```python
from build123d import *

# Parameters (mm, degrees)
ESBO_O1_R                                  = 3
RESSALTO_EXTRUS_O1_DEPTH                   = 1.5
ESBO_O2_R                                  = 2.15
RESSALTO_EXTRUS_O2_DEPTH                   = 6
BROCA_DE_ROSQUEAR_PARA_TARRAXA_DE_M3X0_5_D = 2.5
FILETE1_R                                  = 0.3


with BuildPart() as part:
    # Esboço1 → Ressalto-extrusão1 (new body)
    with BuildSketch(Plane.XY):
        with Locations((-15.341260315, 7.915210608)):
            Circle(ESBO_O1_R)
    extrude(amount=RESSALTO_EXTRUS_O1_DEPTH)

    # Esboço2 → Ressalto-extrusão2 (add)
    with BuildSketch(Plane.XY.offset(1.5)):
        with Locations((-15.341260315, 7.915210608)):
            Circle(ESBO_O2_R)
    extrude(amount=RESSALTO_EXTRUS_O2_DEPTH)

    # Broca de rosquear para tarraxa de M3x0.51 (through all)
    with Locations(Plane(origin=(0, 0, 0), x_dir=(-1, 0, 0), z_dir=(0, 0, -1))):
        with Locations((15.341260315, 7.915210608)):
            Hole(BROCA_DE_ROSQUEAR_PARA_TARRAXA_DE_M3X0_5_D / 2)

    # Filete1
    filete1_edges = [part.edges().sort_by_distance(p)[0] for p in [
        (-17.491260315, 7.915210608, 7.5),
    ]]
    fillet(filete1_edges, radius=FILETE1_R)


solid = part.part
```
The model under review builds one solid part; all positions refer to its coordinate system, in mm. A direction names the side the tool comes from. Round coordinates to 2 decimals unless told otherwise and drop trailing zeros. Loops run counter-clockwise (first coordinate to the right, second up) from the corner with the lowest first, then second, coordinate; pieces in that order, holes last. Notation, with made-up numbers: (-24.5, 84.5) -> (9.5, 84.5) arc R24 ccw to (9.5, 109.5) -> close; hole circle Ø11 at (62, 49). An arc over 180 degrees is marked (long way). Answer as a JSON object with one key per item and string values. Group by question number.
1) We need section B-B on z = 4.75. Write out the cut boundary in (x, y), then the cut area to 3 significant figures.
2) For pin 1 Ø3 at (x, z) = (-15, 3.5) entering from +Y; pin 2 Ø2 at (x, y) = (-15.34, 7.92) entering from -Z; pin 3 Ø1.5 at (x, y) = (-13, 6) entering from -Z; pin 4 Ø3 at (x, z) = (-14.5, 4) entering from -Y, all flat-tipped, find the tip position at first contact; note any pin that passes through.
3) For line 1 (Z direction, x = -14.3, y = 10.05); line 2 (X direction, y = 9, z = 3.5) (3 decimals); line 3 (Y direction, x = -15.95, z = 4.5), list the stretches that pass through material, from the lowest coordinate up. Write a range as [from, to].
4) We need section D-D on z = 1. Write out the cut boundary in (x, y), then the cut area to 3 significant figures.
5) Mouldability with a two-part tool opening along Y and no side actions: class faces 3 (the face through (-16.26, 8.76, 3.8)), 4 (the face through (-14.349, 6.008, 4.31)), 5 (the face through (-14, 7, 0)) as released by +Y, released by -Y, zero draft, split by the parting line, or undercut.
6) For faces 1 (the face through (-13, 7, 1.5)), 2 (the face through (-17, 8, 7.5)), list the 3-axis set-ups (+Z, -Z, +X, -X, +Y, -Y) from which the entire face can be reached by the end or side of a thin tool; tool diameter is ignored.
7) We need section C-C on y = 5.5. Write out the cut boundary in (x, z).
8) We need section A-A on x = -13.1. Write out the cut boundary in (y, z), then the cut area to 3 significant figures.
Result set:
{
 "1": {"outline": "circle Ø4.3 at (-15.34, 7.92); hole circle Ø2.5 at (-15.34, 7.92)", "area": "9.61 mm²"},
 "2": {"pin 1": "y = 10.07", "pin 2": "through", "pin 3": "z = 0", "pin 4": "y = 5.77"},
 "3": {"line 1": "[0, 1.5]", "line 2": "[-17.198, -15.962], [-14.72, -13.485]", "line 3": "[5.85, 6.82], [9.01, 9.98]"},
 "4": {"outline": "circle Ø6 at (-15.34, 7.92); hole circle Ø2.5 at (-15.34, 7.92)", "area": "23.4 mm²"},
 "5": {"face 3": "undercut", "face 4": "split by the parting line", "face 5": "zero draft"},
 "6": {"face 1": "+Z", "face 2": "+Z, +X, -X, +Y, -Y"},
 "7": {"outline": "(-17.12, 0) -> (-13.56, 0) -> (-13.56, 1.5) -> (-17.12, 1.5) -> close"},
 "8": {"outline": "(5.92, 0) -> (9.91, 0) -> (9.91, 1.5) -> (5.92, 1.5) -> close", "area": "5.98 mm²"}
}
